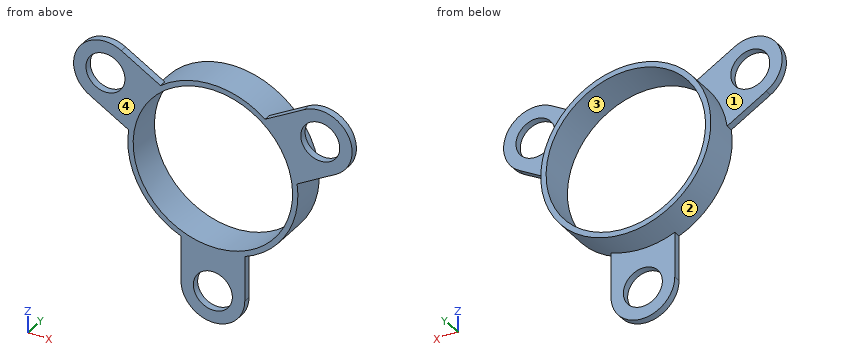
```python
from build123d import *

# Parameters (mm, degrees)
SKETCH1_R             = 2.75
BOSS_EXTRUDE1_DEPTH   = 1
BOSS_EXTRUDE1_2_DEPTH = 1
BOSS_EXTRUDE1_3_DEPTH = 1
SKETCH1_4_R           = 12
SKETCH1_4_R_2         = 11.25
BOSS_EXTRUDE2_DEPTH   = 5


with BuildPart() as part:
    # Sketch1 → Boss-Extrude1 (new body)
    with BuildSketch(Plane(origin=(0, 0, 0), x_dir=(1, 0, 0), z_dir=(0, 1, 0))):
        with BuildLine():
            ThreePointArc((12.905444566, -12.647114317), (19.052558883, -11), (17.405444566, -4.852885683))
            Line((17.405444566, -4.852885683), (11.883924434, -1.665034548))
            ThreePointArc((11.883924434, -1.665034548), (10.392304845, -6), (7.383924434, -9.459263182))
            Line((7.383924434, -9.459263182), (12.905444566, -12.647114317))
        make_face()
        with Locations(Location((15.155444566, -8.75, 0), (0, 0, 270))):
            Circle(SKETCH1_R, mode=Mode.SUBTRACT)
    extrude(amount=BOSS_EXTRUDE1_DEPTH)



with BuildPart() as body_2:
    # Sketch1 → Boss-Extrude1 2 (new body)
    with BuildSketch(Plane(origin=(0, 0, 0), x_dir=(1, 0, 0), z_dir=(0, 1, 0))):
        with BuildLine():
            ThreePointArc((-17.405444566, -4.852885683), (-19.052558883, -11), (-12.905444566, -12.647114317))
            Line((-12.905444566, -12.647114317), (-7.383924434, -9.459263182))
            ThreePointArc((-7.383924434, -9.459263182), (-10.392304845, -6), (-11.883924434, -1.665034548))
            Line((-11.883924434, -1.665034548), (-17.405444566, -4.852885683))
        make_face()
        with Locations(Location((-15.155444566, -8.75, 0), (0, 0, 270))):
            Circle(SKETCH1_R, mode=Mode.SUBTRACT)
    extrude(amount=BOSS_EXTRUDE1_2_DEPTH)


with BuildPart() as body_3:
    # Sketch1 → Boss-Extrude1 3 (new body)
    with BuildSketch(Plane(origin=(0, 0, 0), x_dir=(1, 0, 0), z_dir=(0, 1, 0))):
        with BuildLine():
            ThreePointArc((-4.5, 11.124297731), (0, 12), (4.5, 11.124297731))
            Line((4.5, 11.124297731), (4.5, 17.5))
            ThreePointArc((4.5, 17.5), (0, 22), (-4.5, 17.5))
            Line((-4.5, 17.5), (-4.5, 11.124297731))
        make_face()
        with Locations(Location((0, 17.5, 0), (0, 0, 270))):
            Circle(SKETCH1_R, mode=Mode.SUBTRACT)
    extrude(amount=BOSS_EXTRUDE1_3_DEPTH)


with BuildPart() as part_1:
    add(part.part)

    add(body_2.part)  # Boss-Extrude2 merges body 2

    add(body_3.part)  # Boss-Extrude2 merges body 3
    # Sketch1_4 → Boss-Extrude2 (add)
    with BuildSketch(Plane(origin=(0, 0, 0), x_dir=(1, 0, 0), z_dir=(0, 1, 0))):
        with Locations(Location((0, 0, 0), (0, 0, 67.975687163))):
            Circle(SKETCH1_4_R)
        with Locations(Location((0, 0, 0), (0, 0, 270))):
            Circle(SKETCH1_4_R_2, mode=Mode.SUBTRACT)
    extrude(amount=BOSS_EXTRUDE2_DEPTH)


solid = part_1.part
```
Source: CAD feature listing. Evaluate the final solid. Frame: model axes, mm. Face numbers are marked on the shaded views. A direction names the side the tool comes from. Round coordinates to 2 decimals unless told otherwise and drop trailing zeros. Loops run counter-clockwise (first coordinate to the right, second up) from the corner with the lowest first, then second, coordinate; pieces in that order, holes last. Notation, with made-up numbers: M 60,55.5 L 77,55.5 A22 cw 77,67.5 Z; hole C 56.25,-28.5 d2. An arc over 180 degrees is marked long. Use a Markdown table: item, result. Add a question column.
1. Pull-direction query (Z, two-part tool) for the marked faces 3 and 4; classes: +Z half, -Z half, draft (parallel to the pull), parting line (faces both ways), or undercut.
2. Contact query for flat-ended pins moving along their axis: pin 1 (3 mm diameter, centred on y = 2, z = 5.5, fed in from -X); pin 2 (1 mm diameter, centred on x = -11, y = 2, fed in from -Z); pin 3 (13.5 mm diameter, centred on x = 0, z = 0, fed in from +Y); pin 4 (1.1 mm diameter, centred on y = 0.5, z = -14.5, fed in from -X). Output: stop coordinate, or through.
3. Set-up query: the marked faces 1 and 2. Return all of +Z, -Z, +X, -X, +Y, -Y with unobstructed straight access to the full face (end or side cutting, diameter ignored); none if empty.
4. Cut plane C-C, the plane x = 9. Output: boundary loops of the cut face in (y, z), and give its area (3 significant figures).
5. Cut plane D-D, the plane z = 8.75. Output: boundary loops of the cut face in (x, y).
6. Ray query, line 1 along X through (y, z) = (2.1, 0); line 2 along X through (y, z) = (0.4, -17.5); line 3 along Z through (x, y) = (8.5, 3.55). Return the intervals inside material, ascending. Write a range as [from, to].
7. Cut plane B-B, the plane x = 0. Output: boundary loops of the cut face in (y, z), and give its area (3 significant figures).
8. Cut plane A-A, the plane z = 0. Output: boundary loops of the cut face in (x, y).
Solution:
| question | item | result |
|---|---|---|
| 1 | face 3 | undercut |
| 1 | face 4 | draft |
| 2 | pin 1 | stops at x = -19.12 |
| 2 | pin 2 | stops at z = -5.81 |
| 2 | pin 3 | passes through |
| 2 | pin 4 | stops at x = -4.5 |
| 3 | face 1 | +Z, -X, +Y |
| 3 | face 2 | +Y |
| 4 | outline | M 0,-7.94 L 5,-7.94 L 5,-6.75 L 0,-6.75 Z; M 0,6.75 L 5,6.75 L 5,7.94 L 1,7.94 L 1,10.39 L 0,10.39 Z |
| 4 | area | 14.3 mm2 |
| 5 | outline | M -19.66,0 L -17.91,0 L -17.91,1 L -19.66,1 Z; M -12.41,0 L -7.07,0 L -7.07,5 L -8.21,5 L -8.21,1 L -12.41,1 Z; M 7.07,0 L 12.41,0 L 12.41,1 L 8.21,1 L 8.21,5 L 7.07,5 Z; M 17.91,0 L 19.66,0 L 19.66,1 L 17.91,1 Z |
| 6 | line 1 | x = [-12, -11.25], [11.25, 12] |
| 6 | line 2 | x = [-4.5, -2.75], [2.75, 4.5] |
| 6 | line 3 | z = [-8.47, -7.37], [7.37, 8.47] |
| 7 | outline | M 0,-22 L 1,-22 L 1,-20.25 L 0,-20.25 Z; M 0,-14.75 L 1,-14.75 L 1,-12 L 5,-12 L 5,-11.25 L 0,-11.25 Z; M 0,11.25 L 5,11.25 L 5,12 L 0,12 Z |
| 7 | area | 12.0 mm2 |
| 8 | outline | M -12,0 L -11.25,0 L -11.25,5 L -12,5 Z; M 11.25,0 L 12,0 L 12,5 L 11.25,5 Z |
